Verification items for the finished model (mm, model axes). Face numbers are marked on the shaded views. A direction names the side the tool comes from. Round coordinates to 2 decimals unless told otherwise and drop trailing zeros. Write each loop counter-clockwise with the first axis right and the second up, starting at its lowest first coordinate (ties: lowest second). Pieces come first, ordered by that corner, then holes. Notation, with made-up numbers: M 75,88 L 108,88 A10 cw 108,104 Z; hole C 46,-36 d8. An arc over 180 degrees is marked long. Use a Markdown table: item, result. Add a question column.
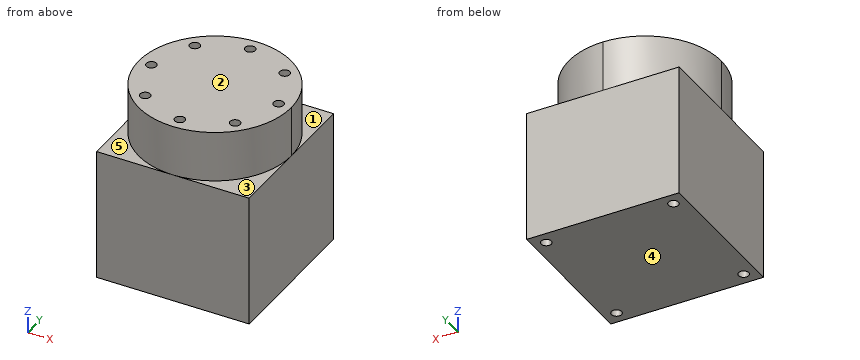
from build123d import *

# Parameters (mm, degrees)
F1_DEPTH = 52
F2_DEPTH = 20
F3_R     = 2
F4_DEPTH = 5
F5_R     = 2
F6_DEPTH = 20


with BuildPart() as f1:
    # F0 (on Top) → F1 (new body)
    with BuildSketch(Plane.XY):
        with BuildLine():
            Line((4.28e-08, 30), (-30, 30))
            Line((-30, 30), (-30, 0))
            ThreePointArc((-30, 0), (-21.2132034204, 21.2132034507), (4.28e-08, 30))
        make_face()
        with BuildLine():
            Line((30, 30), (4.28e-08, 30))
            ThreePointArc((4.28e-08, 30), (21.2132034507, 21.2132034204), (30, 0))
            Line((30, 0), (30, 30))
        make_face()
        with BuildLine():
            ThreePointArc((30, 0), (21.2132034507, 21.2132034204), (4.28e-08, 30))
            ThreePointArc((4.28e-08, 30), (-21.2132034204, 21.2132034507), (-30, 0))
            ThreePointArc((-30, 0), (-21.2132034356, -21.2132034356), (0, -30))
            ThreePointArc((0, -30), (21.2132034356, -21.2132034356), (30, 0))
        make_face()
        with BuildLine():
            ThreePointArc((0, -30), (-21.2132034356, -21.2132034356), (-30, 0))
            Line((-30, 0), (-30, -30))
            Line((-30, -30), (0, -30))
        make_face()
        with BuildLine():
            Line((30, -30), (30, 0))
            ThreePointArc((30, 0), (21.2132034356, -21.2132034356), (0, -30))
            Line((0, -30), (30, -30))
        make_face()
    extrude(amount=-F1_DEPTH)

    # F0 (on Top) → F2 (join)
    with BuildSketch(Plane.XY):
        with BuildLine():
            ThreePointArc((30, 0), (21.2132034507, 21.2132034204), (4.28e-08, 30))
            ThreePointArc((4.28e-08, 30), (-21.2132034204, 21.2132034507), (-30, 0))
            ThreePointArc((-30, 0), (-21.2132034356, -21.2132034356), (0, -30))
            ThreePointArc((0, -30), (21.2132034356, -21.2132034356), (30, 0))
        make_face()
    extrude(amount=F2_DEPTH)

    # F3 (on face) → F4 (cut)
    with BuildSketch(Plane.XY.offset(20)):
        with Locations((0, 25)):
            Circle(F3_R)
        with Locations((-17.6776695297, 17.6776695297)):
            Circle(F3_R)
        with Locations((-25, 0)):
            Circle(F3_R)
        with Locations((-17.6776695297, -17.6776695297)):
            Circle(F3_R)
        with Locations((0, -25)):
            Circle(F3_R)
        with Locations((17.6776695297, -17.6776695297)):
            Circle(F3_R)
        with Locations((25, 0)):
            Circle(F3_R)
        with Locations((17.6776695297, 17.6776695297)):
            Circle(F3_R)
    extrude(amount=-F4_DEPTH, mode=Mode.SUBTRACT)

    # F5 (on face) → F6 (cut)
    with BuildSketch(Plane(origin=(0, 0, -52), x_dir=(1, 0, 0), z_dir=(0, 0, -1))):
        with Locations((-25, 25)):
            Circle(F5_R)
        with Locations((25, -25)):
            Circle(F5_R)
        with Locations((25, 25)):
            Circle(F5_R)
        with Locations((-25, -25)):
            Circle(F5_R)
    extrude(amount=-F6_DEPTH, mode=Mode.SUBTRACT)


solid = f1.part
1. Depth check by flat-ended pin: pin 1 Ø2 at (x, y) = (-24.5, 24.5) entering from -Z; pin 2 Ø6.5 at (x, y) = (-25, 25) entering from +Z; pin 3 Ø1 at (x, z) = (-2, 9) entering from -Y. Enter the tip coordinate at first touch or a pass-through.
2. Scan lines: line 1 along X through (y, z) = (25, -44.5); line 2 along Y through (x, z) = (25, 17.8); line 3 along Z through (x, y) = (-25, -19.5). Record each from-to range of solid material in increasing order. Write a range as from..to.
3. Access from +Z, -Z, +X, -X, +Y, -Y to the whole of each face (thin tool, end or side, straight path). Record for the marked faces 1, 2, 3, 4 and 5.
4. Cross-section at C-C on z = 8.5. Enter the section's corners in (x, y), plus the area to 3 significant figures.
5. Cross-section at A-A on x = -17. Enter the section's corners in (y, z), plus the area to 3 significant figures.
6. Cross-section at B-B on y = -12. Enter the section's corners in (x, z), plus the area to 3 significant figures.
7. Cross-section at D-D on x = 10. Enter the section's corners in (y, z).
Answer:
| question | item | result |
|---|---|---|
| 1 | pin 1 | stops at z = -32 |
| 1 | pin 2 | stops at z = 0 |
| 1 | pin 3 | stops at y = -29.96 |
| 2 | line 1 | x = -30..-27, -23..23, 27..30 |
| 2 | line 2 | y = -16.58..-2, 2..16.58 |
| 2 | line 3 | z = -52..0 |
| 3 | face 1 | +Z, +X, +Y |
| 3 | face 2 | +Z, +X, -X, +Y, -Y |
| 3 | face 3 | +Z, +X, -Y |
| 3 | face 4 | -Z, +X, -X, +Y, -Y |
| 3 | face 5 | +Z, -X, -Y |
| 4 | outline | C 0,0 d60 |
| 4 | area | 2,830 mm^2 |
| 5 | outline | M -30,-52 L 30,-52 L 30,0 L 24.72,0 L 24.72,20 L 19.56,20 L 19.56,15 L 15.8,15 L 15.8,20 L -15.8,20 L -15.8,15 L -19.56,15 L -19.56,20 L -24.72,20 L -24.72,0 L -30,0 Z |
| 5 | area | 4,070 mm^2 |
| 6 | outline | M -30,-52 L 30,-52 L 30,0 L 27.5,0 L 27.5,20 L -27.5,20 L -27.5,0 L -30,0 Z |
| 6 | area | 4,220 mm^2 |
| 7 | outline | M -30,-52 L 30,-52 L 30,0 L 28.28,0 L 28.28,20 L -28.28,20 L -28.28,0 L -30,0 Z |
